Autodesk Inventor part; units mm, degrees
ref_plane "Work Plane1" through (0, 0, -10) normal (0, 0, 1) x (1, 0, 0)
ref_plane "Work Plane3" through (0, 6, -20) normal (0, -1, 0) x (1, 0, 0)
ref_plane "YZ Plane" through (0, 0, 0) normal (1, 0, 0) x (0, 1, 0)
sketch "Sketch1" plane through (0, 0, 0) normal (1, 0, 0) x (0, 1, 0)
  line L0 (0, 0) -> (12, 0)
  line L1 (12, 0) -> (12, -20)
  line L2 (12, -20) -> (0, -20)
  line L3 (0, -20) -> (0, 0)
  circle A0 centre (6, -13) radius 4.5
  dimension "d0" = 20
  dimension "d1" = 12
  dimension "d2" = 6
  dimension "d3" = 13
  dimension "d4" = 9
extrude "Extrusion1" add sketch "Sketch1" against normal blind 50 contours L0 L1 L2 L3 | A0
ref_plane "Work Plane1" through (0, 0, -10) normal (0, 0, 1) x (1, 0, 0)
ref_plane "Work Plane3" through (0, 6, -20) normal (0, -1, 0) x (1, 0, 0)
sketch "Sketch4" plane through (0, 12, 0) normal (0, 1, 0) x (1, 0, 0)
  line L0 (0, 0) -> (0, 20)
  line L1 (0, 0) -> (-50, 0)
  circle A0 centre (-3.5, 3.5) radius 1.6
  dimension "d93" = 3.2
  dimension "d94" = 3.5
  dimension "d95" = 3.5
hole "Hole1" at (0, 6, -13) direction (-1, 0, 0) diameter 9 depth 45
hole "Hole2" at (-3.5, 12, -3.5) direction (0, -1, 0) diameter 3.2 end through all
pattern_linear "Rectangular Pattern7" count 2 spacing 43 along (-1, 0, 0) of "Hole2"
sketch "Sketch2" plane through (0, 0, 0) normal (0, 0, 1) x (1, 0, 0)
  line L0 (0, 0) -> (-50, 0)
  line L1 (0, 0) -> (0, 12)
  circle A0 centre (-10, 6) radius 2.15
  dimension "d7" = 4.3
  dimension "d8" = 6
  dimension "d9" = 10
hole "Hole6" at (-10, 6, 0) direction (0, 0, -1) diameter 4.3 depth 10
pattern_linear "Rectangular Pattern10" count 4 spacing 10 along (-1, 0, 0) of "Hole6"
equation "\"d2\" = 0.5 * d1"
equation "\"d8\" = 0.5 * d1"
properties part number "AirVacManifold_v2"
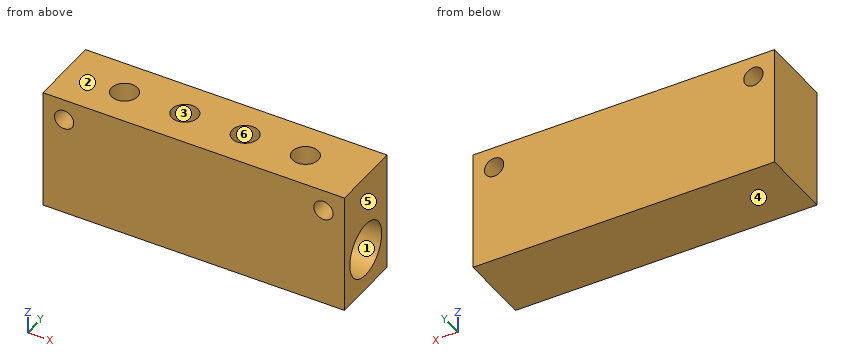
The model under review builds one solid part; all positions refer to its coordinate system, in mm. Face numbers are marked on the shaded views. A direction names the side the tool comes from. Round coordinates to 2 decimals unless told otherwise and drop trailing zeros. Loops run counter-clockwise (first coordinate to the right, second up) from the corner with the lowest first, then second, coordinate; pieces in that order, holes last.
Item 1: Clearance check with flat-ended pins moving along their axes: pin 1 Ø2.5 at (x, y) = (-20, 6) entering from +Z; pin 2 Ø4 at (x, y) = (-10, 6) entering from +Z; pin 3 Ø3 at (x, z) = (-3.5, -3.5) entering from +Y. State where each tip first meets the part, or that it passes through.
Determined:
pin 1: stops at z = -17.32
pin 2: stops at z = -17.03
pin 3: passes through
Item 2: Take a section at A-A (y = 6). Write out the cut boundary in (x, z), then the cut area to 3 significant figures.
Determined:
outline: (-50, -20) - (0, -20) - (0, -17.5) - (-45, -17.5) - (-45, -8.5) - (-42.15, -8.5) - (-42.15, 0) - (-50, 0) - close; (-37.85, -8.5) - (-32.15, -8.5) - (-32.15, 0) - (-37.85, 0) - close; (-27.85, -8.5) - (-22.15, -8.5) - (-22.15, 0) - (-27.85, 0) - close; (-17.85, -8.5) - (-12.15, -8.5) - (-12.15, 0) - (-17.85, 0) - close; (-7.85, -8.5) - (0, -8.5) - (0, 0) - (-7.85, 0) - close; hole circle Ø3.2 at (-46.5, -3.5); hole circle Ø3.2 at (-3.5, -3.5)
area: 433 mm2
Item 3: Take a section at B-B (z = -2.75). Write out the cut boundary in (x, y).
Determined:
outline: (-50, 0) - (-47.91, 0) - (-47.91, 12) - (-50, 12) - close; (-45.09, 0) - (-4.91, 0) - (-4.91, 12) - (-45.09, 12) - close; (-2.09, 0) - (0, 0) - (0, 12) - (-2.09, 12) - close; hole circle Ø4.3 at (-40, 6); hole circle Ø4.3 at (-30, 6); hole circle Ø4.3 at (-20, 6); hole circle Ø4.3 at (-10, 6)
Item 4: For line 1 (X direction, y = 6, z = -6.5); line 2 (Z direction, x = -16, y = 6); line 3 (X direction, y = 6.75, z = -6), list the stretches that pass through material, from the lowest coordinate up.
Determined:
line 1: x = -50 to -42.15, -37.85 to -32.15, -27.85 to -22.15, -17.85 to -12.15, -7.85 to 0
line 2: z = -20 to -17.5, -8.5 to 0
line 3: x = -50 to -42.01, -37.99 to -32.01, -27.99 to -22.01, -17.99 to -12.01, -7.99 to 0
Item 5: For the marked faces 5 and 6, list the 3-axis set-ups (+Z, -Z, +X, -X, +Y, -Y) from which the entire face can be reached by the end or side of a thin tool; tool diameter is ignored.
Determined:
face 5: +Z, -Z, +X, +Y, -Y
face 6: +Z
Item 6: Take a section at C-C (z = -13). Write out the cut boundary in (x, y).
Determined:
outline: (-50, 0) - (0, 0) - (0, 1.5) - (-45, 1.5) - (-45, 10.5) - (0, 10.5) - (0, 12) - (-50, 12) - close
Item 7: Mouldability with a two-part tool opening along Z and no side actions: class the marked faces 1, 2, 3 and 4 as released by +Z, released by -Z, zero draft, split by the parting line, or undercut.
Determined:
face 1: undercut
face 2: released by +Z
face 3: zero draft
face 4: released by -Z
Item 8: Take a section at D-D (x = -30). Write out the cut boundary in (y, z), then the cut area to 3 significant figures.
Determined:
outline: (0, -20) - (12, -20) - (12, 0) - (8.15, 0) - (8.15, -9.05) arc R4.5 cw (long way) to (3.85, -9.05) - (3.85, 0) - (0, 0) - close
area: 139 mm2
